Could you check a few things on this model? Use its own coordinates, in mm. A direction names the side the tool comes from. Give positions to 0.01 mm unless a question says otherwise; leave off trailing zeros. Loops run counter-clockwise (first coordinate to the right, second up) from the corner with the lowest first, then second, coordinate; pieces in that order, holes last.
1. Thinking about a two-plate mould opening in X: for faces 1 (the cylindrical face through (48.48, 85.68, 554.59)), 2 (the flat face through (47, 49, 281)), 3 (the flat face through (50, 49, 281)), which applies, +X half, -X half, draft (parallel to the pull), parting line (faces both ways), or undercut?
2. I need wall thicknesses on line 1 along Y through (x, z) = (10.5, 409.5); line 2 along X through (y, z) = (54.5, 454.5). Which ranges of each line are inside material? Lowest first, please.
3. Imagine slicing it at B-B (x = 21). List the corners of the cut face in (y, z) for me, plus the area to 3 significant figures.
4. Imagine slicing it at C-C (z = 461). List the corners of the cut face in (x, y) for me.
5. For P1, Ø6, axis at y = 14.54, z = 80.53, coming from the +X side; P2, Ø13.5, axis at y = 14.54, z = 559.7, coming from the -X side, each with a flat end and sliding along its axis, tell me the tip position at first contact or that it passes through.
6. Imagine slicing it at A-A (y = 50). List the corners of the cut face in (x, z) for me, plus the area to 3 significant figures.
7. For faces 4 (the cylindrical face through (1.479, 14.765, 484.362)), 5 (the flat face through (25, 3, 281)), which set-ups out of +Z, -Z, +X, -X, +Y, -Y let a thin tool reach every point of the face, with its end or its side?
```python
from build123d import *

# Parameters (mm, degrees)
SKETCH1_W           = 50
SKETCH1_H           = 100
SKETCH1_W_2         = 44
SKETCH1_H_2         = 94
BOSS_EXTRUDE1_DEPTH = 570
SKETCH2_R           = 27.5
CUT_EXTRUDE1_DEPTH  = 570
SKETCH3_R           = 5.115212426
CUT_EXTRUDE2_DEPTH  = 570


with BuildPart() as part:
    # Sketch1 → Boss-Extrude1 (new body)
    with BuildSketch(Plane.XY):
        with Locations((25, 50)):
            Rectangle(SKETCH1_W, SKETCH1_H)
        with Locations((25, 50)):
            Rectangle(SKETCH1_W_2, SKETCH1_H_2, mode=Mode.SUBTRACT)
    extrude(amount=BOSS_EXTRUDE1_DEPTH)

    # Sketch2 → Cut-Extrude1 (cut)
    with BuildSketch(Plane.ZY):
        with Locations((45.413528793, 50)):
            Circle(SKETCH2_R)
        with Locations(Location((524.586471207, 50, 0), (0, 0, 180))):
            Circle(SKETCH2_R)
    extrude(amount=-CUT_EXTRUDE1_DEPTH, mode=Mode.SUBTRACT)

    # Sketch3 → Cut-Extrude2 (cut)
    with BuildSketch(Plane.ZY):
        with Locations((80.527883109, 85.459683227)):
            Circle(SKETCH3_R)
        with Locations((10.299174477, 14.540316773)):
            Circle(SKETCH3_R)
        with Locations((80.527883109, 14.540316773)):
            Circle(SKETCH3_R)
        with Locations((559.700825523, 85.459683227)):
            Circle(SKETCH3_R)
        with Locations((489.472116891, 85.459683227)):
            Circle(SKETCH3_R)
        with Locations((489.472116891, 14.540316773)):
            Circle(SKETCH3_R)
        with Locations((559.700825523, 14.540316773)):
            Circle(SKETCH3_R)
        with Locations((10.299174477, 85.459683227)):
            Circle(SKETCH3_R)
    extrude(amount=-CUT_EXTRUDE2_DEPTH, mode=Mode.SUBTRACT)


solid = part.part
```
Derived:
1. face 1: draft
1. face 2: undercut
1. face 3: +X half
2. line 1: y = 0 to 3, 97 to 100
2. line 2: x = 0 to 3, 47 to 50
3. outline: (0, 0) - (3, 0) - (3, 570) - (0, 570) - close; (97, 0) - (100, 0) - (100, 570) - (97, 570) - close
3. area: 3,420 mm2
4. outline: (0, 0) - (50, 0) - (50, 100) - (0, 100) - close; hole (3, 3) - (47, 3) - (47, 97) - (3, 97) - close
5. P1: passes through
5. P2: stops at x = 0
6. outline: (0, 0) - (3, 0) - (3, 17.91) - (0, 17.91) - close; (0, 72.91) - (3, 72.91) - (3, 497.09) - (0, 497.09) - close; (0, 552.09) - (3, 552.09) - (3, 570) - (0, 570) - close; (47, 0) - (50, 0) - (50, 17.91) - (47, 17.91) - close; (47, 72.91) - (50, 72.91) - (50, 497.09) - (47, 497.09) - close; (47, 552.09) - (50, 552.09) - (50, 570) - (47, 570) - close
6. area: 2,760 mm2
7. face 4: +X, -X
7. face 5: +Z, -Z
